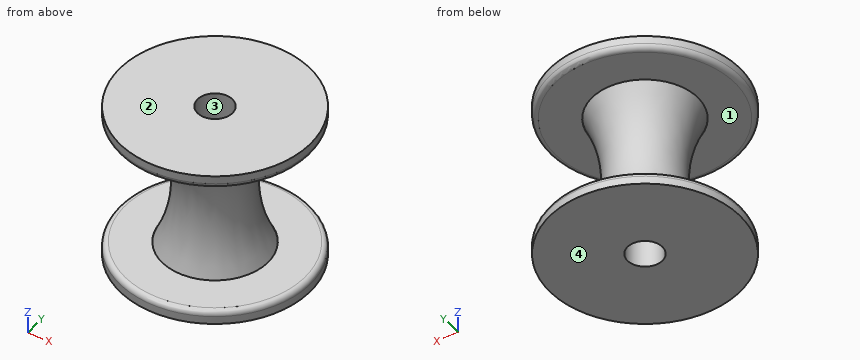
```python
from build123d import *

# Parameters (mm, degrees)
F0_R      = 10
F0_R_2    = 3.3
F1_DEPTH  = 15
F2_DEPTH  = 15
F4_R      = 28
F6_R      = 18
F6_R_2    = 10
F7_DEPTH  = 2.5
F8_R      = 1
F9_R      = 18
F9_R_2    = 10
F10_DEPTH = 2.5
F11_R     = 1


with BuildPart() as f1:
    # F0 (on Top) → F1 (new body)
    with BuildSketch(Plane.XY):
        with Locations((-61.262965, -46.257019)):
            Circle(F0_R)
        with Locations((-61.262965, -46.257019)):
            Circle(F0_R_2, mode=Mode.SUBTRACT)
    extrude(amount=F1_DEPTH)

    # F0 (on Top) → F2 (join)
    with BuildSketch(Plane.XY):
        with Locations((-61.262965, -46.257019)):
            Circle(F0_R)
        with Locations((-61.262965, -46.257019)):
            Circle(F0_R_2, mode=Mode.SUBTRACT)
    extrude(amount=-F2_DEPTH)

    # F5: sweep along a path in F0
    with BuildLine(Plane.XY) as f5_path:
        CenterArc((-61.262965, -46.257019), 10, 0, 360)
    # F4 (on face) → F5 (sweep, cut)
    with BuildSketch(Plane.XZ.offset(46.257019)):
        with Locations((-26.262965, 0)):
            Circle(F4_R)
    sweep(path=f5_path.line, mode=Mode.SUBTRACT)

    # F6 (on face) → F7 (join)
    with BuildSketch(Plane.XY.offset(15)):
        with Locations((-61.262965, -46.257019)):
            Circle(F6_R)
        with Locations((-61.262965, -46.257019)):
            Circle(F6_R_2, mode=Mode.SUBTRACT)
    extrude(amount=-F7_DEPTH)

    # F8
    f8_edges = [f1.edges().sort_by_distance(p)[0] for p in [
        (-79.262965, -46.257019, 12.5),
    ]]
    fillet(f8_edges, radius=F8_R)

    # F9 (on face) → F10 (join)
    with BuildSketch(Plane(origin=(0, 0, -15), x_dir=(1, 0, 0), z_dir=(0, 0, -1))):
        with Locations((-61.262965, 46.257019)):
            Circle(F9_R)
        with Locations((-61.262965, 46.257019)):
            Circle(F9_R_2, mode=Mode.SUBTRACT)
    extrude(amount=-F10_DEPTH)

    # F11
    f11_edges = [f1.edges().sort_by_distance(p)[0] for p in [
        (-79.262965, -46.257019, -12.5),
    ]]
    fillet(f11_edges, radius=F11_R)


solid = f1.part
```
Input: part model. Units: mm. Frame: model coordinates. Face numbers are marked on the shaded views. A direction names the side the tool comes from. Round coordinates to 2 decimals unless told otherwise and drop trailing zeros. Loops run counter-clockwise (first coordinate to the right, second up) from the corner with the lowest first, then second, coordinate; pieces in that order, holes last. Notation, with made-up numbers: (11.25, -36.5) -> (25.25, -36.5) arc R20 ccw to (25.25, -15.5) -> close; hole circle Ø9 at (13.25, 84). An arc over 180 degrees is marked (long way). Use one line per item in the form item = value. Start each with the question number.
Item 1: Section query B-B on z = -12. Return the cut outline in (x, y).
Item 2: Material intervals for L1, parallel to Z at x = -61, y = -61; L2, parallel to X at y = -47, z = 9.75; L3, parallel to Y at x = -61, z = 12.75, sorted ascending. Write a range as from..to.
Item 3: Section query A-A on z = -4. Return the cut outline in (x, y).
Item 4: Contact query for flat-ended pins moving along their axis: pin 1 Ø1 at (y, z) = (-36, -7) entering from +X; pin 2 Ø4 at (x, z) = (-57, 5) entering from +Y; pin 3 Ø5 at (y, z) = (-43.5, -6.5) entering from +X; pin 4 Ø10 at (x, z) = (-59, -4.5) entering from -Y. Output: stop coordinate, or through.
Item 5: Set-up query: the marked faces 1 and 2. Return all of +Z, -Z, +X, -X, +Y, -Y with unobstructed straight access to the full face (end or side cutting, diameter ignored); none if empty.
Item 6: Mould query, pull axis X, two halves, no side actions, for the marked faces 3 and 4. Classes: pulls with the +X half, pulls with the -X half, needs draft (parallel to the pull), parting line crosses it, or undercut.
Ans:
q1.outline = circle Ø19.4 at (-61.26, -46.26); hole circle Ø6.6 at (-61.26, -46.26)
q2.L1 = -15..-12.5, 12.5..15
q2.L2 = -69.98..-64.48, -58.05..-52.54
q2.L3 = -63.92..-49.55, -42.97..-28.6
q3.outline = circle Ø14.57 at (-61.26, -46.26); hole circle Ø6.6 at (-61.26, -46.26)
q4.pin_1 = through
q4.pin_2 = -39.04
q4.pin_3 = -53.03
q4.pin_4 = -54.8
q5.face_1 = none
q5.face_2 = +Z, +X, -X, +Y, -Y
q6.face_3 = undercut
q6.face_4 = needs draft
